Could you check a few things on this model? Use its own coordinates, in mm. A direction names the side the tool comes from. Coordinates: 2 decimals unless noted, no trailing zeros. Order: outer loops, then holes, each group sorted by start corner. A loop starts at its lowest first (then second) coordinate and runs counter-clockwise, first axis right, second up.
```python
from build123d import *

# Parameters (mm, degrees)
SKETCH1_R                       = 13.1
SKETCH1_R_2                     = 2.5
BOSS_EXTRUDE1_DEPTH             = 6
SKETCH2_R                       = 13.7
SKETCH2_R_2                     = 12.7
BOSS_EXTRUDE2_DEPTH             = 8
BOSS_EXTRUDE2_DIRECTION_2_REACH = 21.474
SKETCH7_R                       = 2.5
CUT_EXTRUDE4_DEPTH              = 6


with BuildPart() as part:
    # Sketch1 → Boss-Extrude1 (new body)
    with BuildSketch(Plane(origin=(0, 0, 0), x_dir=(1, 0, 0), z_dir=(0, 1, 0))):
        with Locations(Location((0, 0, 0), (0, 0, 270))):
            Circle(SKETCH1_R)
        with Locations(Location((0, 0, 0), (0, 0, 270))):
            Circle(SKETCH1_R_2, mode=Mode.SUBTRACT)
    extrude(amount=BOSS_EXTRUDE1_DEPTH)

    # Sketch2 → Boss-Extrude2 (add)
    with BuildSketch(Plane(origin=(0, 6, 0), x_dir=(1, 0, 0), z_dir=(0, 1, 0))):
        with Locations(Location((0, 0, 0), (0, 0, 270))):
            Circle(SKETCH2_R)
        with Locations(Location((0, 0, 0), (0, 0, 270))):
            Circle(SKETCH2_R_2, mode=Mode.SUBTRACT)
    extrude(amount=BOSS_EXTRUDE2_DEPTH)

    # Boss-Extrude2 direction 2: up to this face of the body (flat: up to its plane)
    boss_extrude2_direction_2_end = Plane(part.part.faces().sort_by_distance((0, 0, -12.729476047))[0])
    # Sketch2 → Boss-Extrude2 direction 2 (add, up to the picked face)
    with BuildSketch(Plane(origin=(0, 6, 0), x_dir=(1, 0, 0), z_dir=(0, 1, 0)), mode=Mode.PRIVATE) as boss_extrude2_direction_2_sk1:
        with Locations(Location((0, 0, 0), (0, 0, 270))):
            Circle(SKETCH2_R)
        with Locations(Location((0, 0, 0), (0, 0, 270))):
            Circle(SKETCH2_R_2, mode=Mode.SUBTRACT)
    boss_extrude2_direction_2_tool1 = split(extrude(boss_extrude2_direction_2_sk1.sketch, amount=-BOSS_EXTRUDE2_DIRECTION_2_REACH, mode=Mode.PRIVATE), bisect_by=boss_extrude2_direction_2_end, keep=Keep.BOTH, mode=Mode.PRIVATE)
    add(boss_extrude2_direction_2_tool1.solids().sort_by(Axis((0, 6, -13.312505), (0, -1, 0)))[0])

    # Sketch7 → Cut-Extrude4 (cut)
    with BuildSketch(Plane(origin=(0, 6, 0), x_dir=(1, 0, 0), z_dir=(0, 1, 0))):
        with Locations(Location((0, 10, 0), (0, 0, 270))):
            Circle(SKETCH7_R)
        with Locations(Location((8.660254038, 5, 0), (0, 0, 270))):
            Circle(SKETCH7_R)
        with Locations(Location((8.660254038, -5, 0), (0, 0, 270))):
            Circle(SKETCH7_R)
        with Locations(Location((0, -10, 0), (0, 0, 270))):
            Circle(SKETCH7_R)
        with Locations(Location((-8.660254038, -5, 0), (0, 0, 270))):
            Circle(SKETCH7_R)
        with Locations(Location((-8.660254038, 5, 0), (0, 0, 270))):
            Circle(SKETCH7_R)
    extrude(amount=-CUT_EXTRUDE4_DEPTH, mode=Mode.SUBTRACT)


solid = part.part
```
Item 1: Thinking about a two-plate mould opening in Z: for faces 1 (the face through (-7.909, 3.042, 7.385)), 2 (the face through (4.115, 7.098, 13.067)), 3 (the face through (-9.1, 14, 9.1)), which applies, +Z half, -Z half, draft (parallel to the pull), parting line (faces both ways), or undercut?
Item 2: Suppose I cut it at A-A (z = 0). List the corners of the cut face in (x, y) for me.
Item 3: Suppose I cut it at C-C (x = 9). List the corners of the cut face in (y, z) for me, and give its area (3 significant figures).
Item 4: Suppose I cut it at D-D (z = 4). List the corners of the cut face in (x, y) for me.
Item 5: Which directions (+Z, -Z, +X, -X, +Y, -Y) give clear straight access to the entire face, cutting with the end or side of a thin tool? Please do faces 4 (the face through (0.1, 3, 7.5)), 5 (the face through (0, 6, 3)).
Item 6: Suppose I cut it at B-B (x = 0). List the corners of the cut face in (y, z) for me.
Item 7: For pin 1 Ø1.5 at (y, z) = (5.5, 4) entering from +X; pin 2 Ø4 at (x, y) = (8, 9) entering from +Z; pin 3 Ø3 at (y, z) = (12.5, -10.5) entering from -X, each with a flat end and sliding along its axis, tell me the tip position at first contact or that it passes through.
Item 8: I need wall thicknesses on line 1 (X direction, y = 2.25, z = 0); line 2 (X direction, y = 3.75, z = -5) (3 decimals); line 3 (Z direction, x = 10.5, y = 2.5). Which ranges of each line are inside material? Lowest first, please.
Geometry results:
1. face 1: undercut
1. face 2: parting line
1. face 3: draft
2. outline: (-13.7, 0) - (-2.5, 0) - (-2.5, 6) - (-12.7, 6) - (-12.7, 14) - (-13.7, 14) - close; (2.5, 0) - (13.7, 0) - (13.7, 14) - (12.7, 14) - (12.7, 6) - (2.5, 6) - close
3. outline: (0, -10.33) - (14, -10.33) - (14, -8.96) - (6, -8.96) - (6, -7.48) - (0, -7.48) - close; (0, -2.52) - (6, -2.52) - (6, 2.52) - (0, 2.52) - close; (0, 7.48) - (6, 7.48) - (6, 8.96) - (14, 8.96) - (14, 10.33) - (0, 10.33) - close
3. area: 86.4 mm2
4. outline: (-13.1, 0) - (-10.95, 0) - (-10.95, 6) - (-12.05, 6) - (-12.05, 14) - (-13.1, 14) - close; (-6.37, 0) - (6.37, 0) - (6.37, 6) - (-6.37, 6) - close; (10.95, 0) - (13.1, 0) - (13.1, 14) - (12.05, 14) - (12.05, 6) - (10.95, 6) - close
5. face 4: +Y, -Y
5. face 5: +Y
6. outline: (0, -13.7) - (14, -13.7) - (14, -12.7) - (6, -12.7) - (6, -12.5) - (0, -12.5) - close; (0, -7.5) - (6, -7.5) - (6, -2.5) - (0, -2.5) - close; (0, 2.5) - (6, 2.5) - (6, 7.5) - (0, 7.5) - close; (0, 12.5) - (6, 12.5) - (6, 12.7) - (14, 12.7) - (14, 13.7) - (0, 13.7) - close
7. pin 1: stops at x = 13.31
7. pin 2: stops at z = 12.32
7. pin 3: stops at x = -10.33
8. line 1: x = -13.7 to -2.5, 2.5 to 13.7
8. line 2: x = -12.755 to -11.16, -6.16 to 6.16, 11.16 to 12.755
8. line 3: z = -8.8 to -6.69, -3.31 to 3.31, 6.69 to 8.8
